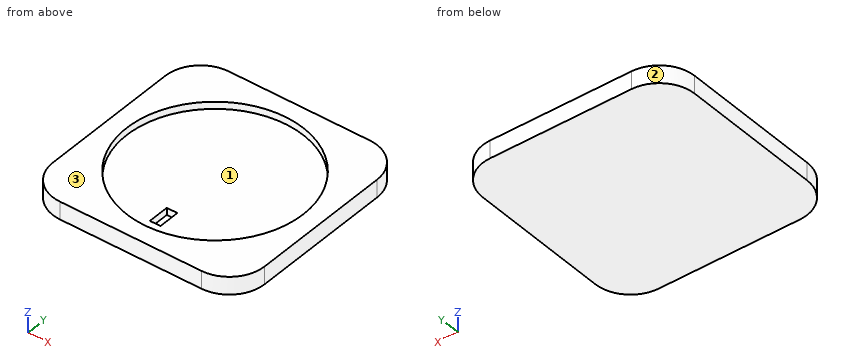
```python
from build123d import *

# Parameters (mm, degrees)
F0_W     = 60
F0_H     = 60
F0_R     = 25
F1_DEPTH = 5
F2_DEPTH = 3
F3_R     = 10
F4_W     = 3
F4_H     = 6
F5_DEPTH = 2


with BuildPart() as f1:
    # F0 (on Top) → F1 (new body)
    with BuildSketch(Plane.XY):
        with Locations((-50.299739, 22.454603)):
            Rectangle(F0_W, F0_H)
        with Locations((-50.299739, 22.454603)):
            Circle(F0_R, mode=Mode.SUBTRACT)
    extrude(amount=F1_DEPTH)

    # F0 (on Top) → F2 (join)
    with BuildSketch(Plane.XY):
        with Locations((-50.299739, 22.454603)):
            Circle(F0_R)
    extrude(amount=F2_DEPTH)

    # F3
    f3_edges = [f1.edges().sort_by_distance(p)[0] for p in [
        (-20.299739, -7.545397, 2.5),
        (-80.299739, -7.545397, 2.5),
        (-80.299739, 52.454603, 2.5),
        (-20.299739, 52.454603, 2.5),
    ]]
    fillet(f3_edges, radius=F3_R)

    # F4 (on face) → F5 (cut)
    with BuildSketch(Plane.XY.offset(3)):
        with Locations((-50.516435, 4.454603)):
            Rectangle(F4_W, F4_H)
    extrude(amount=-F5_DEPTH, mode=Mode.SUBTRACT)


solid = f1.part
```
Source: CAD feature listing. Evaluate the final solid. Frame: model axes, mm. Face numbers are marked on the shaded views. Coordinates: 2 decimals unless noted, no trailing zeros. Loops run counter-clockwise (first coordinate to the right, second up) from the corner with the lowest first, then second, coordinate; pieces in that order, holes last. Notation, with made-up numbers: M -36.75,50 L 0.25,50 A26 ccw 0.25,84 Z; hole C 15.25,43 d2. An arc over 180 degrees is marked long. Put each result on its own line as item: value. Start each with the question number.
1) Ray query, L1, parallel to X at y = 4.5, z = 2.1; L2, parallel to Z at x = -50, y = 40.5; L3, parallel to Y at x = -69.5, z = 3.4. Return the intervals inside material, ascending. Write a range as from..to.
2) Contact query for flat-ended pins moving along their axis: pin 1 Ø2 at (y, z) = (46, 3.5) entering from +X; pin 2 Ø10 at (x, y) = (-68.5, 17.5) entering from +Z; pin 3 Ø1.5 at (x, y) = (-51, 4.5) entering from +Z. Output: stop coordinate, or through.
3) Cut plane B-B on y = 46. Return the cut outline in (x, z).
4) Pull-direction query (Y, two-part tool) for the marked faces 1, 2 and 3; classes: pulls with the +Y half, pulls with the -Y half, needs draft (parallel to the pull), parting line crosses it, or undercut.
5) Cut plane C-C on x = -72. Return the cut outline in (y, z).
6) Cut plane A-A on z = 2.3. Return the cut outline in (x, y).
The answers:
1. L1: x = -80.3..-52.02, -49.02..-20.3
1. L2: z = 0..3
1. L3: y = -7.55..6.44, 38.47..52.45
2. pin 1: stops at x = -20.63
2. pin 2: stops at z = 3
2. pin 3: stops at z = 1
3. outline: M -79.65,0 L -20.95,0 L -20.95,5 L -41.9,5 L -41.9,3 L -58.7,3 L -58.7,5 L -79.65,5 Z
4. face 1: undercut
4. face 2: pulls with the +Y half
4. face 3: needs draft
5. outline: M -7.4,0 L 52.31,0 L 52.31,5 L 34.87,5 L 34.87,3 L 10.04,3 L 10.04,5 L -7.4,5 Z
6. outline: M -80.3,2.45 A10 ccw -70.3,-7.55 L -30.3,-7.55 A10 ccw -20.3,2.45 L -20.3,42.45 A10 ccw -30.3,52.45 L -70.3,52.45 A10 ccw -80.3,42.45 Z; hole M -52.02,1.45 L -49.02,1.45 L -49.02,7.45 L -52.02,7.45 Z
